```python
from build123d import *

# Parameters (mm, degrees)
SKETCH_R          = 2.5
PAD_DEPTH         = 4
SKETCH003_R       = 5
SKETCH003_R_2     = 2.5
PAD001_DEPTH      = 9
SKETCH002_W       = 12.9
SKETCH002_H       = 16.151024
POCKET_DEPTH      = 30.001
POCKET_DEPTH_BACK = 5.001
FILLET_R          = 3
SKETCH004_R       = 5.05
POCKET001_DEPTH   = 1


with BuildPart() as part:
    # Sketch → Pad (new body)
    with BuildSketch(Plane.XY):
        with BuildLine():
            Line((-10, -5), (10, -5))
            ThreePointArc((10, -5), (15, 0), (10, 5))
            Line((7.5, 5), (10, 5))
            Line((7.5, 30), (7.5, 5))
            Line((-7.5, 30), (7.5, 30))
            Line((-29.3, 30), (-7.5, 30))
            Line((-29.3, 20.2), (-29.3, 30))
            Line((-7.5, 20.2), (-29.3, 20.2))
            Line((-7.5, 5), (-7.5, 20.2))
            Line((-7.5, 5), (-10.000009, 5))
            ThreePointArc((-10.000009, 5), (-15, -4e-06), (-10, -5))
        make_face()
        with Locations((-10, 0)):
            Circle(SKETCH_R, mode=Mode.SUBTRACT)
        with Locations((10, 0)):
            Circle(SKETCH_R, mode=Mode.SUBTRACT)
        with Locations((0, 20)):
            Circle(SKETCH_R, mode=Mode.SUBTRACT)
        with Locations((-9.3, 25.2)):
            Circle(SKETCH_R, mode=Mode.SUBTRACT)
        with Locations((-24.3, 25.2)):
            Circle(SKETCH_R, mode=Mode.SUBTRACT)
    extrude(amount=PAD_DEPTH)

    # Sketch003 (on DatumPlane) → Pad001 (join)
    with BuildSketch(Plane.XY.offset(4)):
        with Locations((-10, 0)):
            Circle(SKETCH003_R)
        with Locations((-10, 0)):
            Circle(SKETCH003_R_2, mode=Mode.SUBTRACT)
        with Locations((10, 0)):
            Circle(SKETCH003_R)
        with Locations((10, 0)):
            Circle(SKETCH003_R_2, mode=Mode.SUBTRACT)
    extrude(amount=PAD001_DEPTH)

    # Sketch002 → Pocket (cut, two sides)
    with BuildSketch(Plane.XZ) as pocket_sk:
        with Locations((0, 12.075512)):
            Rectangle(SKETCH002_W, SKETCH002_H)
    extrude(amount=-POCKET_DEPTH, mode=Mode.SUBTRACT)
    extrude(pocket_sk.sketch, amount=POCKET_DEPTH_BACK, mode=Mode.SUBTRACT)

    # Fillet
    fillet_edges = [part.edges().sort_by_distance(p)[0] for p in [
        (-29.3, 20.2, 2),
        (-29.3, 30, 2),
        (-7.5, 20.2, 2),
        (7.5, 30, 2),
    ]]
    fillet(fillet_edges, radius=FILLET_R)

    # Sketch004 (on Face5 of Fillet) → Pocket001 (cut)
    with BuildSketch(Plane.XY.offset(4)):
        with Locations((0, 20)):
            Circle(SKETCH004_R)
    extrude(amount=-POCKET001_DEPTH, mode=Mode.SUBTRACT)


solid = part.part
```
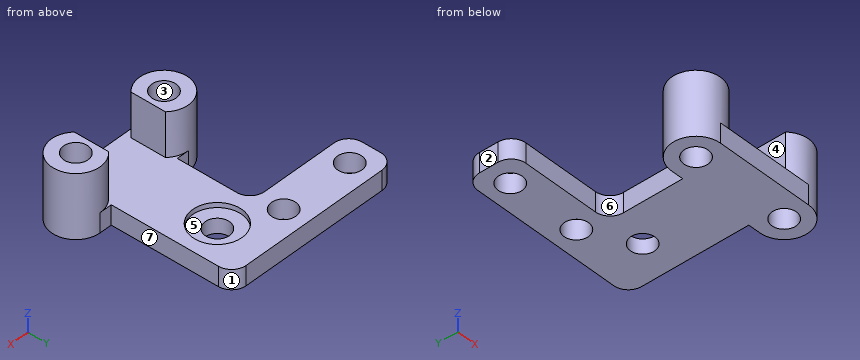
The listing builds one solid part. Answer for the finished solid, in the listing's coordinates (mm). Face numbers are marked on the shaded views. A direction names the side the tool comes from. Coordinates: 2 decimals unless noted, no trailing zeros. Write each loop counter-clockwise with the first axis right and the second up, starting at its lowest first coordinate (ties: lowest second). Pieces come first, ordered by that corner, then holes. Notation, with made-up numbers: M 44.25,-15.75 L 90.25,-15.75 A8 cw 90.25,-9.75 Z; hole C 4.5,36 d1. An arc over 180 degrees is marked long. Use a Markdown table: item, result. Add a question column.
1. Section A-A (x = 0) is taken. Give the vertices of the cut face in (y, z).
2. Which of the six approach directions +Z, -Z, +X, -X, +Y, -Y give full straight-line access (tool end or side, diameter ignored) to the marked faces 4, 5, 6 and 7?
3. Section C-C (y = 0) is taken. Give the vertices of the cut face in (x, z), plus the area to 3 significant figures.
4. Given P1, Ø3, axis at x = -9.3, y = 25.2, coming from the +Z side; P2, Ø2, axis at y = -0.5, z = 7.5, coming from the -X side; P3, Ø6, axis at x = -9, z = 10.5, coming from the +Y side; P4, Ø8, axis at x = 0, y = 20, coming from the -Z side, each flat-ended and moving along its own axis, determine where each tip first touches the part or whether it passes through.
5. Straight lines are drawn through the part: line 1 along Y through (x, z) = (-10, 5.75); line 2 along Z through (x, y) = (-3, 17.5); line 3 along Z through (x, y) = (2.5, 5). For each, find the intervals that lie inside material, in ascending order. Write a range as [from, to].
6. Section D-D (z = 1) is taken. Give the vertices of the cut face in (x, y).
7. For a pull along X with two mould halves and no side action, classify the marked faces 1, 2 and 3 as +X half, -X half, draft (parallel to the pull), parting line (faces both ways), or undercut.
8. Section B-B (z = 10.25) is taken. Give the vertices of the cut face in (x, y).
Data:
| question | item | result |
|---|---|---|
| 1 | outline | M -5,0 L 17.5,0 L 17.5,3 L 14.95,3 L 14.95,4 L -5,4 Z; M 22.5,0 L 30,0 L 30,4 L 25.05,4 L 25.05,3 L 22.5,3 Z |
| 2 | face 4 | +Z, +Y, -Y |
| 2 | face 5 | +Z |
| 2 | face 6 | +Z, -Z, -X |
| 2 | face 7 | +Z, -Z, +X, +Y |
| 3 | outline | M -15,0 L -12.5,0 L -12.5,13 L -15,13 Z; M -7.5,0 L 7.5,0 L 7.5,13 L 6.45,13 L 6.45,4 L -6.45,4 L -6.45,13 L -7.5,13 Z; M 12.5,0 L 15,0 L 15,13 L 12.5,13 Z |
| 3 | area | 144 mm2 |
| 4 | P1 | passes through |
| 4 | P2 | stops at x = -15 |
| 4 | P3 | stops at y = 5 |
| 4 | P4 | stops at z = 0 |
| 5 | line 1 | y = [-5, -2.5], [2.5, 5] |
| 5 | line 2 | z = [0, 3] |
| 5 | line 3 | z = [0, 4] |
| 6 | outline | M -29.3,23.2 A3 ccw -26.3,20.2 L -10.5,20.2 A3 cw -7.5,17.2 L -7.5,5 L -10,5 A5 ccw -10,-5 L 10,-5 A5 ccw 10,5 L 7.5,5 L 7.5,27 A3 ccw 4.5,30 L -26.3,30 A3 ccw -29.3,27 Z; hole C -24.3,25.2 d5; hole C -10,0 d5; hole C -9.3,25.2 d5; hole C 0,20 d5; hole C 10,0 d5 |
| 7 | face 1 | +X half |
| 7 | face 2 | -X half |
| 7 | face 3 | undercut |
| 8 | outline | M -6.45,-3.52 L -6.45,3.52 A5 ccw long Z; M 6.45,-3.52 A5 ccw long 6.45,3.52 Z; hole C -10,0 d5; hole C 10,0 d5 |
